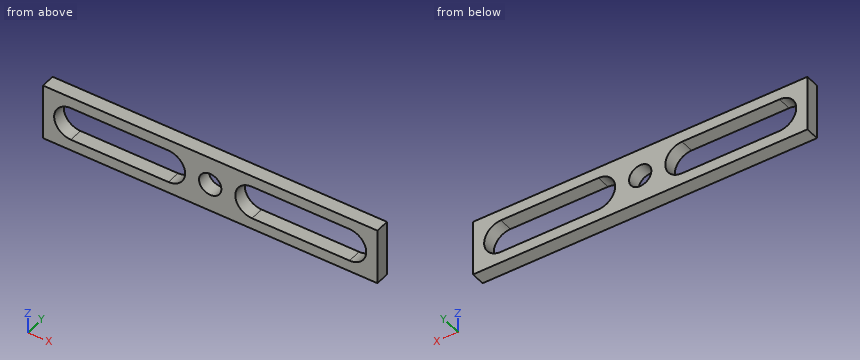
from build123d import *

# Parameters (mm, degrees)
SKETCH1_W           = 76.2
SKETCH1_H           = 12.7
BOSS_EXTRUDE1_DEPTH = 3.175
SKETCH2_R           = 2.54
CUT_EXTRUDE1_DEPTH  = 39.75581408
CUT_EXTRUDE2_DEPTH  = 39.75581408


with BuildPart() as part:
    # Sketch1 → Boss-Extrude1 (new body)
    with BuildSketch(Plane(origin=(0, 0, 0), x_dir=(1, 0, 0), z_dir=(0, 1, 0))):
        Rectangle(SKETCH1_W, SKETCH1_H)
    extrude(amount=BOSS_EXTRUDE1_DEPTH)

    # Sketch2 → Cut-Extrude1 (cut, through all)
    with BuildSketch(Plane(origin=(0, 3.175, 0), x_dir=(1, 0, 0), z_dir=(0, 1, 0))):
        with Locations(Location((0, 0, 0), (0, 0, 270))):
            Circle(SKETCH2_R)
    extrude(amount=-CUT_EXTRUDE1_DEPTH, mode=Mode.SUBTRACT)

    # Sketch4 → Cut-Extrude2 (cut, through all)
    with BuildSketch(Plane(origin=(0, 3.175, 0), x_dir=(1, 0, 0), z_dir=(0, 1, 0))):
        with BuildLine():
            Line((-31.75, 3.81), (-9.525, 3.81))
            ThreePointArc((-9.525, 3.81), (-5.715, 0), (-9.525, -3.81))
            Line((-9.525, -3.81), (-31.75, -3.81))
            ThreePointArc((-31.75, -3.81), (-35.56, 0), (-31.75, 3.81))
        make_face()
        with BuildLine():
            Line((9.525, 3.81), (31.75, 3.81))
            ThreePointArc((31.75, 3.81), (35.56, 0), (31.75, -3.81))
            Line((31.75, -3.81), (9.525, -3.81))
            ThreePointArc((9.525, -3.81), (5.715, 0), (9.525, 3.81))
        make_face()
    extrude(amount=-CUT_EXTRUDE2_DEPTH, mode=Mode.SUBTRACT)


solid = part.part
The listing builds one solid part. Answer for the finished solid, in the listing's coordinates (mm). Round coordinates to 2 decimals unless told otherwise and drop trailing zeros. Write each loop counter-clockwise with the first axis right and the second up, starting at its lowest first coordinate (ties: lowest second). Pieces come first, ordered by that corner, then holes. Notation, with made-up numbers: M 42.5,19 L 84.5,19 A15 ccw 84.5,48 Z; hole C 82,87 d11. An arc over 180 degrees is marked long. Write each question's results on one line, items separated by ' | '. Start each with the question number.
Item 1: Find section A-A on z = 0. Write down the section's boundary in (x, y) (3 decimals).
Item 2: Find section B-B on x = -17.5. Write down the section's boundary in (y, z) (3 decimals).
Item 3: Straight lines are drawn through the part: probe 1 along X at (y, z) = (1.2, 0) (3 decimals); probe 2 along Z at (x, y) = (14, 0.9); probe 3 along X at (y, z) = (1.65, 3). For each, find the intervals that lie inside material, in ascending order.
Item 4: Find section C-C on y = 0.65. Write down the section's boundary in (x, z) (3 decimals).
Answer block:
1) outline: M -38.1,0 L -35.56,0 L -35.56,3.175 L -38.1,3.175 Z; M -5.715,0 L -2.54,0 L -2.54,3.175 L -5.715,3.175 Z; M 2.54,0 L 5.715,0 L 5.715,3.175 L 2.54,3.175 Z; M 35.56,0 L 38.1,0 L 38.1,3.175 L 35.56,3.175 Z
2) outline: M 0,-6.35 L 3.175,-6.35 L 3.175,-3.81 L 0,-3.81 Z; M 0,3.81 L 3.175,3.81 L 3.175,6.35 L 0,6.35 Z
3) probe 1: x = -38.1 to -35.56, -5.715 to -2.54, 2.54 to 5.715, 35.56 to 38.1 | probe 2: z = -6.35 to -3.81, 3.81 to 6.35 | probe 3: x = -38.1 to -34.1, -7.18 to 7.18, 34.1 to 38.1
4) outline: M -38.1,-6.35 L 38.1,-6.35 L 38.1,6.35 L -38.1,6.35 Z; hole M -31.75,-3.81 L -9.525,-3.81 A3.81 ccw -9.525,3.81 L -31.75,3.81 A3.81 ccw Z; hole C 0,0 d5.08; hole M 9.525,-3.81 L 31.75,-3.81 A3.81 ccw 31.75,3.81 L 9.525,3.81 A3.81 ccw Z
